Job drawing, mm, ordinate dimensions from the low corner. One solid piece. Give positions to 0.01 mm unless a question says otherwise; leave off trailing zeros. Order: outer loops, then holes, each group sorted by start corner. A loop starts at its lowest first (then second) coordinate and runs counter-clockwise, first axis right, second up. Notation, with made-up numbers: M 1,66.25 L 16,66.25 A36 ccw 16,100.25 Z; hole C -23.75,36.25 d9. An arc over 180 degrees is marked long. One line per question, with ' | ' between items.
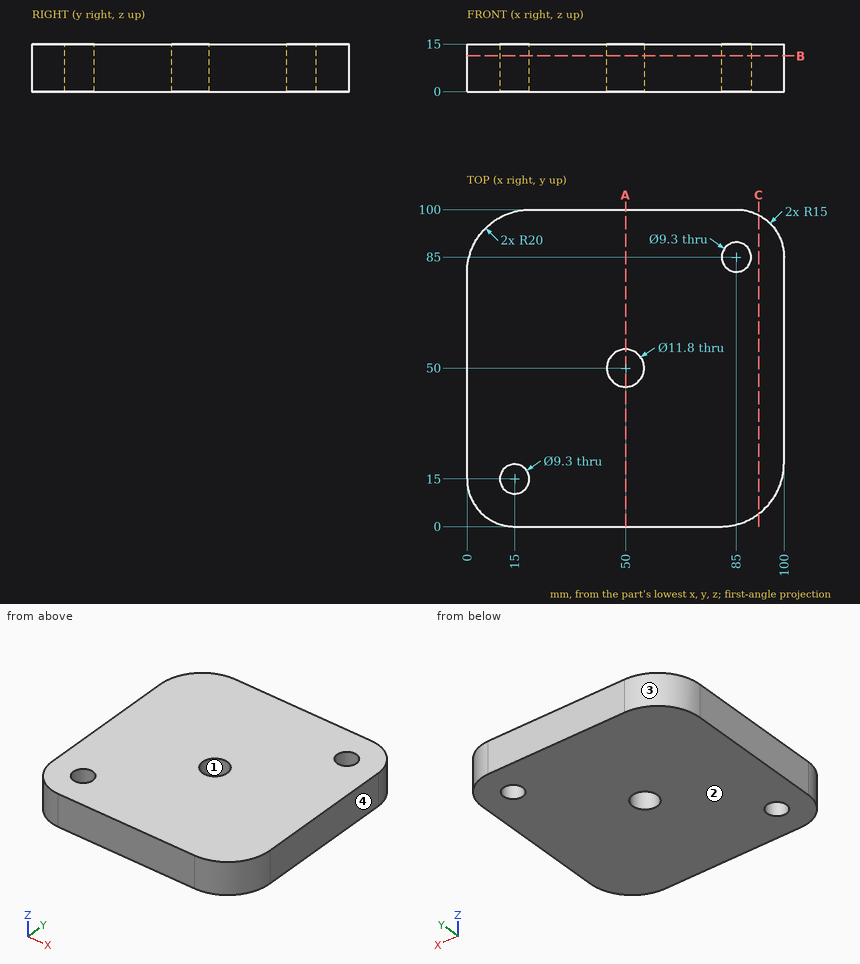
1. Mould opens along X. For the marked faces 1, 2, 3 and 4 say: released by +X, released by -X, zero draft, split by the parting line, or undercut.
Worked out:
face 1: undercut | face 2: zero draft | face 3: released by -X | face 4: released by +X
2. Slice it at C-C on x = 92. Give the cut face in (y, z), then the cut area to 3 significant figures.
Worked out:
outline: M 4,0 L 98.27,0 L 98.27,15 L 4,15 Z | area: 1,410 mm2
3. Drop flat-ended pins along their axis: pin 1 (6 mm diameter, centred on y = 88.5, z = 13.5, fed in from -X); pin 2 (8.5 mm diameter, centred on x = 15, y = 15, fed in from +Z). Give the stop position or say it passes through.
Worked out:
pin 1: stops at x = 0.77 | pin 2: passes through
4. Probe L1, parallel to Y at x = 50, z = 11.25; L2, parallel to X at y = 15, z = 6.75; L3, parallel to X at y = 83.5, z = 10.5. List the from-to ranges inside material, lowest first. Write a range as from..to.
Worked out:
L1: y = 0..44.1, 55.9..100 | L2: x = 0..10.35, 19.65..99.36 | L3: x = 0.31..80.6, 89.4..100
5. Slice it at B-B on z = 11.25. Give the cut face in (x, y).
Worked out:
outline: M 0,15 A15 ccw 15,0 L 80,0 A20 ccw 100,20 L 100,85 A15 ccw 85,100 L 20,100 A20 ccw 0,80 Z; hole C 15,15 d9.3; hole C 50,50 d11.8; hole C 85,85 d9.3
6. Slice it at A-A on x = 50. Give the cut face in (y, z), then the cut area to 3 significant figures.
Worked out:
outline: M 0,0 L 44.1,0 L 44.1,15 L 0,15 Z; M 55.9,0 L 100,0 L 100,15 L 55.9,15 Z | area: 1,320 mm2
